Part model, mm, in its own coordinate system. A direction names the side the tool comes from. Give positions to 0.01 mm unless a question says otherwise; leave off trailing zeros. Loops run counter-clockwise (first coordinate to the right, second up) from the corner with the lowest first, then second, coordinate; pieces in that order, holes last. Notation, with made-up numbers: M -23.75,-11.75 L -4.75,-11.75 A25 cw -4.75,1.25 Z; hole C 67.5,27.25 d6. An arc over 180 degrees is marked long. Answer in a Markdown table with one row per item.
from build123d import *

# Parameters (mm, degrees)
SKETCH1_W           = 29.9085
SKETCH1_H           = 29.9085
BOSS_EXTRUDE1_DEPTH = 6.35
SKETCH2_W           = 33.02
SKETCH2_H           = 33.02
BOSS_EXTRUDE2_DEPTH = 1.4605
SKETCH4_W           = 7.9375
SKETCH4_H           = 7.9375
CUT_EXTRUDE2_DEPTH  = 13.7


with BuildPart() as part:
    # Sketch1 → Boss-Extrude1 (new body, symmetric)
    with BuildSketch(Plane(origin=(0, 0, 0), x_dir=(1, 0, 0), z_dir=(0, 1, 0))):
        Rectangle(SKETCH1_W, SKETCH1_H)
    extrude(amount=BOSS_EXTRUDE1_DEPTH, both=True)

    # Sketch2 → Boss-Extrude2 (add, symmetric)
    with BuildSketch(Plane(origin=(0, 0, 0), x_dir=(1, 0, 0), z_dir=(0, 1, 0))):
        Rectangle(SKETCH2_W, SKETCH2_H)
    extrude(amount=BOSS_EXTRUDE2_DEPTH, both=True)

    # Sketch4 → Cut-Extrude2 (cut, through all)
    with BuildSketch(Plane(origin=(0, 6.35, 0), x_dir=(1, 0, 0), z_dir=(0, 1, 0))):
        Rectangle(SKETCH4_W, SKETCH4_H)
    extrude(amount=-CUT_EXTRUDE2_DEPTH, mode=Mode.SUBTRACT)


solid = part.part
(1) Saw through at C-C (x = -3). Write the cut outline in (y, z), plus the area to 3 significant figures.
Recorded:
| item | result |
|---|---|
| outline | M -6.35,-14.95 L -1.46,-14.95 L -1.46,-16.51 L 1.46,-16.51 L 1.46,-14.95 L 6.35,-14.95 L 6.35,-3.97 L -6.35,-3.97 Z; M -6.35,3.97 L 6.35,3.97 L 6.35,14.95 L 1.46,14.95 L 1.46,16.51 L -1.46,16.51 L -1.46,14.95 L -6.35,14.95 Z |
| area | 288 mm^2 |
(2) Pull direction X, two halves, no side cores. Call faces 1 (the face through (-14.954, 4, 0)), 2 (the face through (0, -4, 14.954)), 3 (the face through (16.51, 0, 0)), 4 (the face through (0, 0, 3.969)): +X half, -X half, draft (parallel to the pull), parting line (faces both ways), or undercut.
Recorded:
| item | result |
|---|---|
| face 1 | -X half |
| face 2 | draft |
| face 3 | +X half |
| face 4 | undercut |
(3) Saw through at D-D (z = -8). Write the cut outline in (x, y), plus the area to 3 significant figures.
Recorded:
| item | result |
|---|---|
| outline | M -16.51,-1.46 L -14.95,-1.46 L -14.95,-6.35 L 14.95,-6.35 L 14.95,-1.46 L 16.51,-1.46 L 16.51,1.46 L 14.95,1.46 L 14.95,6.35 L -14.95,6.35 L -14.95,1.46 L -16.51,1.46 Z |
| area | 389 mm^2 |
(4) Which spindle directions (+Z, -Z, +X, -X, +Y, -Y) get a long thin tool onto all of the face, cutting with end or side? Do faces 5 (the face through (0, -4, -14.954)), 6 (the face through (0, 4, -14.954)), 7 (the face through (0, 4, 14.954)). Say none if no direction does.
Recorded:
| item | result |
|---|---|
| face 5 | -Z, +X, -X, -Y |
| face 6 | -Z, +X, -X, +Y |
| face 7 | +Z, +X, -X, +Y |
(5) Drill centre lines: line 1 along X through (y, z) = (-4.25, -3.5); line 2 along Z through (x, y) = (1, 0.25). Where is each one in solid material? Low to high.
Recorded:
| item | result |
|---|---|
| line 1 | x = -14.95 to -3.97, 3.97 to 14.95 |
| line 2 | z = -16.51 to -3.97, 3.97 to 16.51 |
(6) Saw through at A-A (z = -3). Write the cut outline in (x, y).
Recorded:
| item | result |
|---|---|
| outline | M -16.51,-1.46 L -14.95,-1.46 L -14.95,-6.35 L -3.97,-6.35 L -3.97,6.35 L -14.95,6.35 L -14.95,1.46 L -16.51,1.46 Z; M 3.97,-6.35 L 14.95,-6.35 L 14.95,-1.46 L 16.51,-1.46 L 16.51,1.46 L 14.95,1.46 L 14.95,6.35 L 3.97,6.35 Z |
(7) Saw through at B-B (y = 0.25). Write the cut outline in (x, z), plus the area to 3 significant figures.
Recorded:
| item | result |
|---|---|
| outline | M -16.51,-16.51 L 16.51,-16.51 L 16.51,16.51 L -16.51,16.51 Z; hole M -3.97,-3.97 L 3.97,-3.97 L 3.97,3.97 L -3.97,3.97 Z |
| area | 1,030 mm^2 |
(8) Pin check, flat tips, straight feed: pin 1 Ø1 at (x, y) = (7.5, -4.5) entering from +Z; pin 2 Ø5.5 at (y, z) = (-4.5, 6) entering from -X; pin 3 Ø2.5 at (x, y) = (-5, 3.5) entering from -Z. Stop position of each tip, or through.
Recorded:
| item | result |
|---|---|
| pin 1 | stops at z = 14.95 |
| pin 2 | stops at x = -14.95 |
| pin 3 | stops at z = -14.95 |
